Input: part model. Units: mm. Frame: model coordinates. Coordinates: 2 decimals unless noted, no trailing zeros. Loops run counter-clockwise (first coordinate to the right, second up) from the corner with the lowest first, then second, coordinate; pieces in that order, holes last. Notation, with made-up numbers: (49, 2) -> (90, 2) arc R18 ccw to (90, 23) -> close; hole circle Ø10 at (39, 85). An arc over 180 degrees is marked (long way). Put each result on its own line as item: value. Start each with the question number.
1) Cut plane A-A (z = 4.1). Return the cut outline in (x, y).
2) Contact query for a flat-ended pin moving along its axis: P1, Ø4, axis at x = 79, y = 11, coming from the -Z side. Output: stop coordinate, or through.
3) Cut plane C-C (x = 24). Return the cut outline in (y, z).
4) Material intervals for L1, parallel to Y at x = 50, z = 2.3; L2, parallel to X at y = 65, z = 1.9; L3, parallel to X at y = 80, z = 3.75, sorted ascending.
5) Cut plane B-B (y = 35). Return the cut outline in (x, z), plus the area to 3 significant figures.
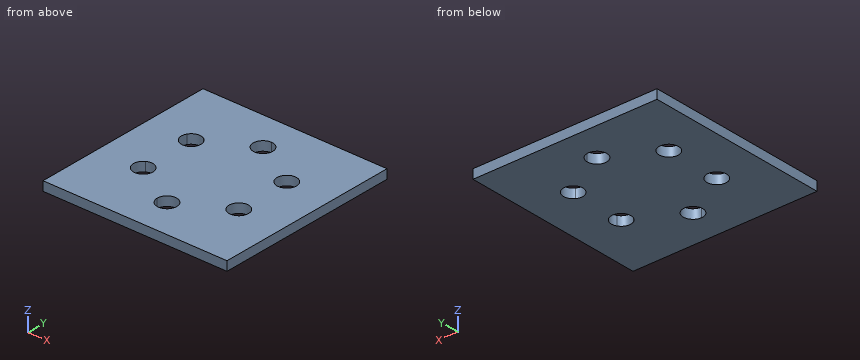
from build123d import *

# Parameters (mm, degrees)
F0_W            = 100
F0_H            = 100
F1_DEPTH        = 5
F3_DEPTH        = 25
F3_COPIES_COUNT = 6


# Not quite as in the source:
# - a pattern or mirror of a feature is missing from the dataset's text; its kind, count and spacing are read off the source's solid


with BuildPart() as f1:
    # F0 (on Top) → F1 (new body)
    with BuildSketch(Plane.XY):
        with Locations((50, 50)):
            Rectangle(F0_W, F0_H)
    extrude(amount=F1_DEPTH)

    # F2 (on face) → F3 (cut)
    with BuildSketch(Plane.XY.offset(5)):
        with BuildLine():
            ThreePointArc((50, 85.3), (46.2523340597, 76.2523340597), (55.3, 80))
            ThreePointArc((55.3, 80), (53.7476659403, 83.7476659403), (50, 85.3))
        make_face()
    f3 = extrude(amount=-F3_DEPTH, mode=Mode.SUBTRACT)

    # F3_copies: F3 ×6 about axis
    f3_copies_axis = Axis((50, 50, 0), (0, 0, 1))
    for i in range(1, F3_COPIES_COUNT):
        add(f3.rotate(f3_copies_axis, i * 360 / F3_COPIES_COUNT), mode=Mode.SUBTRACT)


solid = f1.part
Results found:
1. outline: (0, 0) -> (100, 0) -> (100, 100) -> (0, 100) -> close; hole circle Ø10.6 at (24.02, 35); hole circle Ø10.6 at (24.02, 65); hole circle Ø10.6 at (50, 20); hole circle Ø10.6 at (50, 80); hole circle Ø10.6 at (75.98, 35); hole circle Ø10.6 at (75.98, 65)
2. P1: stops at z = 0
3. outline: (0, 0) -> (29.7, 0) -> (29.7, 5) -> (0, 5) -> close; (40.3, 0) -> (59.7, 0) -> (59.7, 5) -> (40.3, 5) -> close; (70.3, 0) -> (100, 0) -> (100, 5) -> (70.3, 5) -> close
4. L1: y = 0 to 14.7, 25.3 to 74.7, 85.3 to 100
4. L2: x = 0 to 18.72, 29.32 to 70.68, 81.28 to 100
4. L3: x = 0 to 44.7, 55.3 to 100
5. outline: (0, 0) -> (18.72, 0) -> (18.72, 5) -> (0, 5) -> close; (29.32, 0) -> (70.68, 0) -> (70.68, 5) -> (29.32, 5) -> close; (81.28, 0) -> (100, 0) -> (100, 5) -> (81.28, 5) -> close
5. area: 394 mm2
